```python
from build123d import *

# Parameters (mm, degrees)
F0_W    = 4
F0_H    = 8
F0_H_2  = 10
F0_H_3  = 6
F2_SIZE = 2


with BuildPart() as f1:
    # F0 (on Top) → F1 (revolve)
    with BuildSketch(Plane.XY):
        Polygon((49, 0), (24, 0), (24, -8), (24, -13.5), (49, -13.5), (49, -11.5), (53, -11.5), (53, 0), align=None)
        Polygon((63, 0), (53, 0), (53, -11.5), (53, -13.5), (53, -16), (63, -16), (63, -10), align=None)
        with Locations((22, -4)):
            Rectangle(F0_W, F0_H)
        with Locations((65, -5)):
            Rectangle(F0_W, F0_H_2)
        Polygon((88, 0), (67, 0), (67, -10), (67, -12), (88, -12), (88, -6), align=None)
        with Locations((90, -3)):
            Rectangle(F0_W, F0_H_3)
        Polygon((20, 0), (0.5, 0), (0, -0.5), (0, -10), (20, -10), (20, -8), align=None)
        Polygon((112.5, 0), (92, 0), (92, -6), (92, -8), (113, -8), (113, -0.5), align=None)
    revolve(axis=Axis((10, 0, 0), (1, 0, 0)))

    # F2
    f2_edges = [f1.edges().sort_by_distance(p)[0] for p in [
        (0, 10, 0),
        (24, 13.5, 0),
        (53, 16, 0),
        (63, 16, 0),
        (88, 12, 0),
        (113, 8, 0),
    ]]
    chamfer(f2_edges, length=F2_SIZE)


solid = f1.part
```
Geometry: final body of the model. Coordinates: model frame, mm. A direction names the side the tool comes from. Coordinates: 2 decimals unless noted, no trailing zeros. Order: outer loops, then holes, each group sorted by start corner. A loop starts at its lowest first (then second) coordinate and runs counter-clockwise, first axis right, second up. Notation, with made-up numbers: (58, 81) -> (76, 81) arc R17 cw to (76, 92) -> close; hole circle Ø1 at (12, 88). An arc over 180 degrees is marked (long way). Write each question's results on one line, items separated by ' | '. Start each with the question number.
1) First-contact query: pin 1 (5 mm diameter, centred on x = 99, z = -4, fed in from -Y); pin 2 (1.5 mm diameter, centred on x = 98.5, y = 2, fed in from -Z); pin 3 (10 mm diameter, centred on x = 81.5, z = 3.5, fed in from -Y). Flat tips, straight axial feed; report the tip coordinate or a pass-through.
2) Material intervals for line 1 along X through (y, z) = (-3, -13.5); line 2 along X through (y, z) = (-2.5, -8); line 3 along X through (y, z) = (-13, 1), sorted ascending.
3) Mould query, pull axis X, two halves, no side actions, for faces 6 (the cylindrical face through (22.03, 1.73, 7.81)), 7 (the cylindrical face through (11.13, 2.17, 9.76)), 8 (the flat face through (92, -2, -6)), 9 (the conical face through (0.13, 1.06, -8.06)). Classes: released by +X, released by -X, zero draft, split by the parting line, or undercut.
4) Cut plane A-A, the plane x = 29. Output: boundary loops of the cut face in (y, z), and give its area (3 significant figures).
5) Set-up query: faces 1 (the flat face through (24, -8, 2)), 2 (the cylindrical face through (101.63, 1.73, 7.81)), 3 (the cylindrical face through (58.04, 3.47, 15.62)), 4 (the cylindrical face through (37.66, 2.93, 13.18)), 5 (the flat face through (0, 0, 2)). Return all of +Z, -Z, +X, -X, +Y, -Y with unobstructed straight access to the full face (end or side cutting, diameter ignored); none if empty.
Checks:
1) pin 1: y = -7.86 | pin 2: z = -7.9 | pin 3: y = -12
2) line 1: 53 to 63 | line 2: 0.38 to 20, 24 to 88 | line 3: 25.54 to 49, 53 to 63
3) face 6: undercut | face 7: zero draft | face 8: undercut | face 9: released by -X
4) outline: circle Ø27 at (0, 0) | area: 573 mm^2
5) face 1: none | face 2: +X | face 3: +X, -X | face 4: -X | face 5: +Z, -Z, -X, +Y, -Y
